Autodesk Inventor part; units mm, degrees
ref_plane "YZ Plane" through (0, 0, 0) normal (1, 0, 0) x (0, 1, 0)
ref_plane "XZ Plane" through (0, 0, 0) normal (0, 1, 0) x (-1, 0, 0)
ref_plane "XY Plane" through (0, 0, 0) normal (0, 0, 1) x (1, 0, 0)
sketch "Sketch1" plane through (0, 0, 0) normal (0, 0, 1) x (1, 0, 0)
  line L0 (3.6662, 6.35) -> (7.3323, 0)
  line L1 (7.3323, 0) -> (3.6662, -6.35)
  line L2 (3.6662, -6.35) -> (-3.6662, -6.35)
  line L3 (-3.6662, -6.35) -> (-7.3323, 0)
  line L4 (-7.3323, 0) -> (-3.6662, 6.35)
  line L5 (-3.6662, 6.35) -> (3.6662, 6.35)
  point P0 (0, 0)
  point P1 (0, 0)
  dimension "d0" = 12.7
extrude "Extrusion1" add sketch "Sketch1" along normal blind 152.4
sketch "Sketch4" plane through (0, 0, 152.4) normal (0, 0, 1) x (1, 0, 0)
  circle A0 centre (0, 0) radius 2.4384
  dimension "d10" = 4.8768
extrude "Extrusion4" cut sketch "Sketch4" against normal blind 12.7
sketch "Sketch5" plane through (0, 0, 0) normal (0, 0, -1) x (-1, 0, 0)
  circle A0 centre (0, 0) radius 2.4384
  dimension "d13" = 4.8768
extrude "Extrusion5" cut sketch "Sketch5" against normal blind 12.7
properties part number "OuterAxle" material "Aluminum-6061"
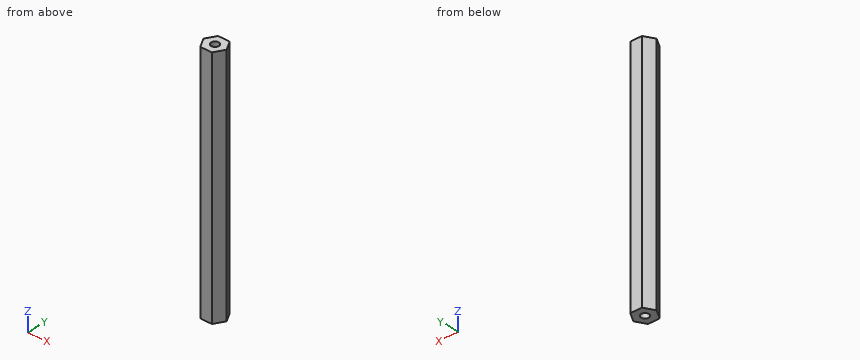
For this review, take the finished solid that the model builds, in its own axes (mm). Coordinates: 2 decimals unless noted, no trailing zeros. Write each loop counter-clockwise with the first axis right and the second up, starting at its lowest first coordinate (ties: lowest second). Pieces come first, ordered by that corner, then holes.
(1) Wall thickness on probe 1 along Y at (x, z) = (0, 145); probe 2 along Y at (x, z) = (-6.25, 12); probe 3 along X at (y, z) = (-5.5, 88): over which ranges is each line inside the solid? List them lowest first.
(2) Add section C-C on y = 5. Give the boundary of the cut face in (x, z).
(3) Add section A-A on z = 130. Give the boundary of the cut face in (x, y).
(4) For pin 1 Ø1.5 at (y, z) = (2, 80.5) entering from +X; pin 2 Ø4 at (x, y) = (0, 0) entering from -Z; pin 3 Ø5 at (y, z) = (3.5, 91.5) entering from -X, all flat-tipped, find the tip position at first contact; note any pin that passes through.
(5) Add section B-B on x = 0. Give the boundary of the cut face in (y, z), then the cut area to 3 significant figures.
Answer sheet:
1. probe 1: y = -6.35 to -2.44, 2.44 to 6.35
1. probe 2: y = -1.87 to 1.87
1. probe 3: x = -4.16 to 4.16
2. outline: (-4.45, 0) - (4.45, 0) - (4.45, 152.4) - (-4.45, 152.4) - close
3. outline: (-7.33, 0) - (-3.67, -6.35) - (3.67, -6.35) - (7.33, 0) - (3.67, 6.35) - (-3.67, 6.35) - close
4. pin 1: stops at x = 6.61
4. pin 2: stops at z = 12.7
4. pin 3: stops at x = -6.75
5. outline: (-6.35, 0) - (-2.44, 0) - (-2.44, 12.7) - (2.44, 12.7) - (2.44, 0) - (6.35, 0) - (6.35, 152.4) - (2.44, 152.4) - (2.44, 139.7) - (-2.44, 139.7) - (-2.44, 152.4) - (-6.35, 152.4) - close
5. area: 1,810 mm2
